from build123d import *

# Parameters (mm, degrees)
F0_W     = 30.75
F0_H     = 13.3
F0_W_2   = 16.25
F0_H_2   = 8.7
F0_W_3   = 11.5
F0_H_3   = 8.8
F1_DEPTH = 10
F2_R     = 0.5
F3_R     = 2
F4_R     = 1.5
F7_DEPTH = 2.5
F5_R     = 1.75
F8_DEPTH = 8


with BuildPart() as f1:
    # F0 (on Top) → F1 (new body)
    with BuildSketch(Plane.XY):
        with Locations((-14.5149128214, -8.8939947993)):
            Rectangle(F0_W, F0_H)
        with Locations((-20.7649128214, -10.0939947993)):
            Rectangle(F0_W_2, F0_H_2, mode=Mode.SUBTRACT)
        with Locations((-5.8899128214, -10.1439947993)):
            Rectangle(F0_W_3, F0_H_3, mode=Mode.SUBTRACT)
    extrude(amount=F1_DEPTH)

    # F2
    f2_edges = [f1.edges().sort_by_distance(p)[0] for p in [
        (-28.889913, -5.743995, 5),
        (-28.889913, -14.443995, 5),
        (-12.639913, -5.743995, 5),
        (-12.639913, -14.443995, 5),
    ]]
    fillet(f2_edges, radius=F2_R)

    # F3
    f3_edges = [f1.edges().sort_by_distance(p)[0] for p in [
        (-0.139913, -5.743995, 5),
        (-0.139913, -14.543995, 5),
        (-11.639913, -14.543995, 5),
        (-11.639913, -5.743995, 5),
    ]]
    fillet(f3_edges, radius=F3_R)

    # F4
    f4_edges = [f1.edges().sort_by_distance(p)[0] for p in [
        (-29.889913, -15.543995, 5),
        (-29.889913, -2.243995, 5),
        (0.860087, -15.543995, 5),
        (0.860087, -2.243995, 5),
    ]]
    fillet(f4_edges, radius=F4_R)

    # F6 (on face) → F7 (cut)
    with BuildSketch(Plane.XZ.offset(5.7439947993)):
        Polygon((-8.8899128214, 6.7320508076), (-8.8899128214, 3.2679491924), (-5.8899128214, 1.5358983849), (-2.8899128214, 3.2679491924), (-2.8899128214, 6.7320508076), (-5.8899128214, 8.4641016151), align=None)
        Polygon((-23.7399128214, 6.7320508076), (-23.7399128214, 3.2679491924), (-20.7399128214, 1.5358983849), (-17.7399128214, 3.2679491924), (-17.7399128214, 6.7320508076), (-20.7399128214, 8.4641016151), align=None)
    extrude(amount=-F7_DEPTH, mode=Mode.SUBTRACT)

    # F5 (on face) → F8 (cut)
    with BuildSketch(Plane(origin=(0, -2.2439947993, 0), x_dir=(-1, 0, 0), z_dir=(0, 1, 0))):
        with Locations((5.8899128214, 5)):
            Circle(F5_R)
        with Locations((20.7399128214, 5)):
            Circle(F5_R)
    extrude(amount=-F8_DEPTH, mode=Mode.SUBTRACT)


solid = f1.part
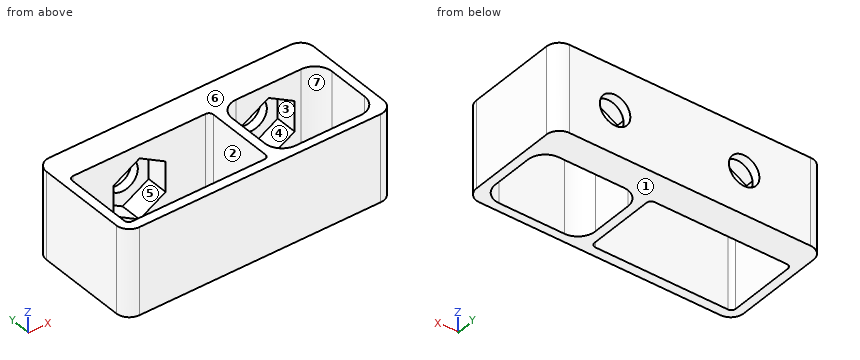
Geometry check sheet. Reference: the model listing, model coordinates, mm. Face numbers are marked on the shaded views. A direction names the side the tool comes from. Give positions to 0.01 mm unless a question says otherwise; leave off trailing zeros. Loops run counter-clockwise (first coordinate to the right, second up) from the corner with the lowest first, then second, coordinate; pieces in that order, holes last. Notation, with made-up numbers: M 71.25,40 L 76.25,40 A18 ccw 76.25,68 Z; hole C 69.5,-38.5 d5. An arc over 180 degrees is marked long. Write each question's results on one line, items separated by ' | '.
1) Section check D-D, the plane x = -4.5. Record the boundary of the cut face in (y, z), plus the area to 3 significant figures.
Answers follow:
outline: M -15.54,0 L -14.54,0 L -14.54,10 L -15.54,10 Z; M -5.74,0 L -2.24,0 L -2.24,3.94 L -3.24,3.94 L -3.24,2.34 L -5.74,2.34 Z; M -5.74,7.66 L -3.24,7.66 L -3.24,6.06 L -2.24,6.06 L -2.24,10 L -5.74,10 Z | area: 29.6 mm2
2) Thickness scan on line 1 (X direction, y = -8.25, z = 8.25); line 2 (Y direction, x = -14.5, z = 1); line 3 (Y direction, x = -3, z = 4.25). Record the ranges inside material, lowest first.
Answers follow:
line 1: -29.89 to -28.89, -12.64 to -11.64, -0.14 to 0.86 | line 2: -15.54 to -14.44, -5.74 to -2.24 | line 3: -15.54 to -14.54, -3.24 to -2.24
3) Release check for a two-part mould opening along Z. For the marked faces 4, 5, 6 and 7 record: +Z half, -Z half, draft (parallel to the pull), parting line (faces both ways), or undercut.
Answers follow:
face 4: undercut | face 5: undercut | face 6: +Z half | face 7: draft
4) Section check C-C, the plane z = 1. Record the boundary of the cut face in (x, y).
Answers follow:
outline: M -29.89,-14.04 A1.5 ccw -28.39,-15.54 L -0.64,-15.54 A1.5 ccw 0.86,-14.04 L 0.86,-3.74 A1.5 ccw -0.64,-2.24 L -28.39,-2.24 A1.5 ccw -29.89,-3.74 Z; hole M -28.89,-13.94 A0.5 ccw -28.39,-14.44 L -13.14,-14.44 A0.5 ccw -12.64,-13.94 L -12.64,-6.24 A0.5 ccw -13.14,-5.74 L -28.39,-5.74 A0.5 ccw -28.89,-6.24 Z; hole M -11.64,-12.54 A2 ccw -9.64,-14.54 L -2.14,-14.54 A2 ccw -0.14,-12.54 L -0.14,-7.74 A2 ccw -2.14,-5.74 L -9.64,-5.74 A2 ccw -11.64,-7.74 Z
5) Section check B-B, the plane x = -8. Record the boundary of the cut face in (y, z).
Answers follow:
outline: M -15.54,0 L -14.54,0 L -14.54,10 L -15.54,10 Z; M -5.74,0 L -2.24,0 L -2.24,10 L -5.74,10 L -5.74,7.25 L -3.24,7.25 L -3.24,2.75 L -5.74,2.75 Z
6) Tool access check on the marked faces 1, 2 and 3. Record the directions out of +Z, -Z, +X, -X, +Y, -Y that give a thin tool (end or side, any length) a straight path to the whole face; none if there is none.
Answers follow:
face 1: -Z, +X, -X, +Y, -Y | face 2: +Z, -Z | face 3: none
7) Section check A-A, the plane y = -8.5. Record the boundary of the cut face in (x, z).
Answers follow:
outline: M -29.89,0 L -28.89,0 L -28.89,10 L -29.89,10 Z; M -12.64,0 L -11.64,0 L -11.64,10 L -12.64,10 Z; M -0.14,0 L 0.86,0 L 0.86,10 L -0.14,10 Z
